Autodesk Inventor part; units mm, degrees
ref_plane "Work Plane2" through (0, 0, 74) normal (0, 0, 1) x (1, 0, 0)
ref_plane "Work Plane3" through (0, 0, 43) normal (0, 0, 1) x (1, 0, 0)
ref_plane "Work Plane6" through (0, 0, 16) normal (0, 0, 1) x (1, 0, 0)
sketch "Sketch1" plane through (0, 0, 0) normal (0, 0, 1) x (1, 0, 0)
  line L0 (-0.2363, 14.3955) -> (15.4637, 14.3955)
  line L1 (15.4637, 14.3955) -> (15.4637, 17.3955)
  line L2 (15.4637, 17.3955) -> (-0.2363, 17.3955)
  line L3 (-0.2363, 17.3955) -> (-0.2363, 14.3955)
  line L4 (15.4637, 14.3955) -> (18.4637, 14.3955)
  line L5 (18.4637, 14.3955) -> (18.4637, -1.3045)
  line L6 (18.4637, -1.3045) -> (15.4637, -1.3045)
  line L7 (15.4637, -1.3045) -> (15.4637, 14.3955)
  line L8 (15.4637, 14.3955) -> (18.4637, 14.3955)
  line L9 (18.4637, 14.3955) -> (18.4637, 17.3955)
  line L10 (18.4637, 17.3955) -> (15.4637, 17.3955)
  line L11 (15.4637, 17.3955) -> (15.4637, 14.3955)
  circle A0 centre (11.9637, 10.8955) radius 2.25
  line L12 (15.4637, 14.3955) -> (8.4637, 14.3955)
  line L13 (8.4637, 14.3955) -> (8.4637, 7.3955)
  line L14 (8.4637, 7.3955) -> (15.4637, 7.3955)
  line L15 (15.4637, 7.3955) -> (15.4637, 14.3955)
  point P0 (0, 0)
  point P1 (11.9637, 7.3955)
  point P2 (8.4637, 10.8955)
  dimension "d2" = 3
  dimension "d3" = 3
  dimension "d9" = 4.5
  dimension "d46" = 7
  dimension "d47" = 7
  dimension "d48" = 15.7
  dimension "d49" = 15.7
extrude "Extrusion1" add sketch "Sketch1" along normal blind 83 contours L3 L2 L1 L0 | L1 L10 L9 L4 | L4 L5 L6 L7
extrude "Extrusion2" add sketch "Sketch1" along normal blind 1.5 contours L0 L7 L14 L13
fillet "Fillet1" radius 3 1 edges at (8.4637, 7.3955, 0.75)
sketch "Sketch3" plane through (-0.2363, 14.3955, 83) normal (0, -1, 0) x (1, 0, 0)
  line L0 (15.7, 0) -> (15.7, -81.5)
  line L1 (0, 0) -> (15.7, 0)
  line L2 (0, -83) -> (0, 0)
  circle A0 centre (6.25, -4) radius 2.25
  line L3 (18.7, -83) -> (0, -83)
  line L4 (0, 0) -> (15.7, 0)
  line L5 (18.7, 0) -> (0, 0)
  line L6 (12.5, 0) -> (12.5, -83) construction
  line L7 (0, -83) -> (0, 0)
  line L8 (12.5, 0) -> (0, 0)
  line L9 (0, -83) -> (8.7, -83)
  line L10 (8.7, -81.5) -> (15.7, -81.5)
  line L11 (8.7, -83) -> (8.7, -81.5)
  point P0 (0.2363, -83)
  point P1 (1.7, -20)
  point P2 (6.25, 0)
  dimension "d12" = 4.5
  dimension "d13" = 4
  dimension "d24" = 12.5
sketch "Sketch4" plane through (15.4637, -1.3045, 83) normal (-1, 0, 0) x (0, 0, 1)
  line L0 (-83, 0) -> (0, 0)
  line L1 (0, 15.7) -> (0, 0)
  line L2 (0, 15.7) -> (-81.5, 15.7)
  circle A0 centre (-4, 6.25) radius 2.25
  line L3 (0, 15.7) -> (0, 0)
  line L4 (-83, 0) -> (-83, 18.7)
  line L5 (0, 15.7) -> (-81.5, 15.7)
  line L6 (0, 12.5) -> (-83, 12.5) construction
  line L7 (0, 12.5) -> (0, 0)
  line L8 (-83, 8.7) -> (-83, 0)
  line L9 (-81.5, 15.7) -> (-81.5, 8.7)
  line L10 (-81.5, 8.7) -> (-83, 8.7)
  point P0 (-83, 1.3045)
  point P1 (-20, 1.7)
  point P2 (0, 6.25)
  point P3 (-83, 15.7)
  dimension "d14" = 4.5
  dimension "d15" = 4
  dimension "d25" = 12.5
extrude "Extrusion4" cut sketch "Sketch3" against normal blind 5 contours A0
extrude "Extrusion5" cut sketch "Sketch4" against normal blind 5 contours A0
sketch "Sketch5" plane through (0, 0, 0) normal (0, 0, 1) x (1, 0, 0)
  line L0 (29.2522, 21.8201) -> (22.8883, 28.184)
  line L1 (22.8883, 28.184) -> (12.2817, 17.5774)
  line L2 (12.2817, 17.5774) -> (18.6456, 11.2135)
  line L3 (18.6456, 11.2135) -> (29.2522, 21.8201)
  line L4 (26.0703, 25.0021) -> (15.4637, 14.3955) construction
  line L5 (23.9489, 16.5168) -> (17.585, 22.8807) construction
  line L6 (15.4637, -1.3045) -> (15.4637, 14.3955)
  line L7 (15.4637, 17.3955) -> (-0.2363, 17.3955)
  line L8 (18.4637, 14.3955) -> (18.4637, -1.3045)
  line L9 (18.4637, 14.3955) -> (18.4637, 17.3955)
  line L10 (18.4637, 17.3955) -> (15.4637, 17.3955)
  circle A0 centre (23.2418, 22.1736) radius 2.25
  line L11 (18.0923, 10.6601) -> (18.6456, 11.2135)
  line L12 (18.6456, 11.2135) -> (12.2817, 17.5774)
  line L13 (12.2817, 17.5774) -> (11.7283, 17.0241)
  line L14 (11.7283, 17.0241) -> (18.0923, 10.6601)
  point P0 (0, 0)
  dimension "d29" = 9
  dimension "d30" = 4.5
  dimension "d31" = 4
  dimension "d32" = 15
  dimension "d56" = 9
extrude "Extrusion6" add sketch "Sketch5" along normal blind 1.5
fillet "Fillet2" radius 2 2 edges at (22.8883, 28.184, 0.75) (29.2522, 21.8201, 0.75)
ref_plane "Work Plane2" through (0, 0, 74) normal (0, 0, 1) x (1, 0, 0)
sketch "Sketch6" plane through (0, 0, 74) normal (0, 0, 1) x (1, 0, 0)
  line L0 (18.4637, -1.3045) -> (18.4637, 17.3955)
  line L1 (18.4637, 17.3955) -> (-0.2363, 17.3955)
  line L2 (-0.2363, 17.3955) -> (-0.2363, 14.3955)
  line L3 (15.4637, -1.3045) -> (18.4637, -1.3045)
  line L4 (-0.2363, 17.3955) -> (-0.2363, 14.3955)
  line L5 (-0.2363, 17.3955) -> (8.4637, 17.3955)
  line L6 (8.4637, 17.3955) -> (8.4637, 14.3955)
  line L7 (8.4637, 14.3955) -> (-0.2363, 14.3955)
  line L8 (-0.2363, 14.3955) -> (-0.2363, 17.3955)
  line L9 (18.4637, -1.3045) -> (15.4637, -1.3045)
  line L10 (15.4637, -1.3045) -> (15.4637, 7.3955)
  line L11 (15.4637, 7.3955) -> (18.4637, 7.3955)
  line L12 (18.4637, 7.3955) -> (18.4637, -1.3045)
  point P0 (0, 0)
  dimension "d45" = 8.7
  dimension "d50" = 7
  dimension "d51" = 7
extrude "Extrusion7" cut sketch "Sketch6" against normal blind 74
ref_plane "Work Plane3" through (0, 0, 43) normal (0, 0, 1) x (1, 0, 0)
ref_plane "Work Plane5" through (0, 0, 39) normal (0, 0, 1) x (1, 0, 0)
sketch "Sketch9" plane through (0, 0, 39) normal (0, 0, 1) x (1, 0, 0)
  line L0 (18.4637, 7.3955) -> (11.4637, 7.3955)
  arc A0 (8.4637, 10.3955) -> (11.4637, 7.3955) centre (11.4637, 10.3955) ccw
  line L1 (8.4637, 10.3955) -> (8.4637, 17.3955)
  line L2 (12.0997, 17.3955) -> (8.4637, 17.3955)
  line L3 (21.4741, 26.7698) -> (12.0997, 17.3955)
  arc A1 (24.3025, 26.7698) -> (21.4741, 26.7698) centre (22.8883, 25.3556) ccw
  line L4 (27.838, 23.2343) -> (24.3025, 26.7698)
  arc A2 (27.838, 20.4059) -> (27.838, 23.2343) centre (26.4238, 21.8201) ccw
  line L5 (18.4637, 11.0315) -> (27.838, 20.4059)
  line L6 (18.4637, 7.3955) -> (18.4637, 11.0315)
  circle A3 centre (23.2418, 22.1736) radius 2.25
  circle A4 centre (11.9637, 10.8955) radius 2.25
  line L7 (12.0997, 17.3955) -> (16.4707, 15.4026)
  line L8 (16.4707, 15.4026) -> (18.4637, 11.0315)
  point P0 (0, 0)
extrude "Extrusion9" add sketch "Sketch9" along normal blind 1.5 contours L8 L7 L3 A1 L4 A2 L5
ref_plane "Work Plane6" through (0, 0, 16) normal (0, 0, 1) x (1, 0, 0)
sketch "Sketch10" plane through (0, 0, 16) normal (0, 0, 1) x (1, 0, 0)
  line L0 (18.4637, 7.3955) -> (11.4637, 7.3955)
  arc A0 (8.4637, 10.3955) -> (11.4637, 7.3955) centre (11.4637, 10.3955) ccw
  line L1 (8.4637, 10.3955) -> (8.4637, 17.3955)
  line L2 (12.0997, 17.3955) -> (8.4637, 17.3955)
  line L3 (21.4741, 26.7698) -> (12.0997, 17.3955)
  arc A1 (24.3025, 26.7698) -> (21.4741, 26.7698) centre (22.8883, 25.3556) ccw
  line L4 (27.838, 23.2343) -> (24.3025, 26.7698)
  arc A2 (27.838, 20.4059) -> (27.838, 23.2343) centre (26.4238, 21.8201) ccw
  line L5 (18.4637, 11.0315) -> (27.838, 20.4059)
  line L6 (18.4637, 7.3955) -> (18.4637, 11.0315)
  circle A3 centre (23.2418, 22.1736) radius 2.25
  circle A4 centre (11.9637, 10.8955) radius 2.25
  line L7 (12.0997, 17.3955) -> (18.4637, 17.3955)
  line L8 (12.0997, 17.3955) -> (16.7869, 15.7187)
  line L9 (18.4637, 17.3955) -> (18.4637, 11.0315)
  line L10 (16.7869, 15.7187) -> (18.4637, 11.0315)
  point P0 (0, 0)
extrude "Extrusion10" add sketch "Sketch10" along normal blind 1.5 contours L9 L7 L3 A1 L4 A2 L5
pattern_linear "Rectangular Pattern2" count 4 spacing 22 along (0, 0, 1) of "Extrusion2", "Fillet1"
ref_plane "Work Plane7" through (0, 0, 63) normal (0, 0, 1) x (1, 0, 0)
sketch "Sketch11" plane through (0, 0, 63) normal (0, 0, 1) x (1, 0, 0)
  arc A0 (27.838, 20.4059) -> (27.838, 23.2343) centre (26.4238, 21.8201) ccw
  line L0 (18.4637, 7.3955) -> (11.4637, 7.3955)
  arc A1 (8.4637, 10.3955) -> (11.4637, 7.3955) centre (11.4637, 10.3955) ccw
  line L1 (8.4637, 10.3955) -> (8.4637, 17.3955)
  line L2 (12.0997, 17.3955) -> (8.4637, 17.3955)
  line L3 (21.4741, 26.7698) -> (12.0997, 17.3955)
  arc A2 (24.3025, 26.7698) -> (21.4741, 26.7698) centre (22.8883, 25.3556) ccw
  line L4 (27.838, 23.2343) -> (24.3025, 26.7698)
  arc A3 (27.838, 20.4059) -> (27.838, 23.2343) centre (26.4238, 21.8201) ccw
  line L5 (18.4637, 11.0315) -> (27.838, 20.4059)
  line L6 (18.4637, 7.3955) -> (18.4637, 11.0315)
  circle A4 centre (23.2418, 22.1736) radius 2.25
  circle A5 centre (11.9637, 10.8955) radius 2.25
  line L7 (18.4637, 11.0315) -> (16.7869, 15.7187)
  line L8 (16.7869, 15.7187) -> (12.0997, 17.3955)
  point P0 (0, 0)
extrude "Extrusion11" add sketch "Sketch11" along normal blind 1.5 contours L5 L7 L8 L3 A2 L4 A0
properties part number "VerticalConnector"
Verification items for the finished model (mm, model axes). A direction names the side the tool comes from. Give positions to 0.01 mm unless a question says otherwise; leave off trailing zeros. Order: outer loops, then holes, each group sorted by start corner. A loop starts at its lowest first (then second) coordinate and runs counter-clockwise, first axis right, second up. Notation, with made-up numbers: (10, -35) -> (30, -35) arc R27 cw to (30, -19) -> close; hole circle Ø6 at (41, 59). An arc over 180 degrees is marked (long way). Use a Markdown table: item, result.
1) Material ranges on probe 1 along Z at (x, y) = (21.5, 19.25); probe 2 along Z at (x, y) = (8.75, 11); probe 3 along X at (y, z) = (14.75, 49), recorded low to high.
Results:
| item | result |
|---|---|
| probe 1 | 0 to 1.5, 16 to 17.5, 39 to 40.5, 63 to 64.5 |
| probe 2 | 0 to 1.5, 22 to 23.5, 44 to 45.5, 66 to 67.5 |
| probe 3 | 8.46 to 18.46 |
2) Section check C-C, the plane y = 25.5. Record the boundary of the cut face in (x, z).
Results:
| item | result |
|---|---|
| outline | (20.2, 0) -> (25.57, 0) -> (25.57, 1.5) -> (20.2, 1.5) -> close; (20.2, 16) -> (25.57, 16) -> (25.57, 17.5) -> (20.2, 17.5) -> close; (20.2, 39) -> (25.57, 39) -> (25.57, 40.5) -> (20.2, 40.5) -> close; (20.2, 63) -> (25.57, 63) -> (25.57, 64.5) -> (20.2, 64.5) -> close |
3) Section check D-D, the plane z = 50.5. Record the boundary of the cut face in (x, y).
Results:
| item | result |
|---|---|
| outline | (8.46, 14.4) -> (15.46, 14.4) -> (15.46, 7.4) -> (18.46, 7.4) -> (18.46, 17.4) -> (8.46, 17.4) -> close |
4) Tool access check on faces 3 (the flat face through (12, 14.396, 34)), 4 (the flat face through (26.09, 24.98, 0.74)). Record the directions out of +Z, -Z, +X, -X, +Y, -Y that give a thin tool (end or side, any length) a straight path to the whole face; none if there is none.
Results:
| item | result |
|---|---|
| face 3 | -X, -Y |
| face 4 | +Z, -Z, +X, +Y |
5) Section check B-B, the plane x = 20.25. Record the boundary of the cut face in (y, z).
Results:
| item | result |
|---|---|
| outline | (12.82, 0) -> (25.55, 0) -> (25.55, 1.5) -> (12.82, 1.5) -> close; (12.82, 16) -> (25.55, 16) -> (25.55, 17.5) -> (12.82, 17.5) -> close; (12.82, 39) -> (25.55, 39) -> (25.55, 40.5) -> (12.82, 40.5) -> close; (12.82, 63) -> (25.55, 63) -> (25.55, 64.5) -> (12.82, 64.5) -> close |
6) Mould release check, pull along Z, two halves, no side actions. Record for faces 1 (the flat face through (23.085, 15.653, 16.74)), 2 (the flat face through (11.9, 13.3, 23.5)): pulls with the +Z half, pulls with the -Z half, needs draft (parallel to the pull), parting line crosses it, or undercut.
Results:
| item | result |
|---|---|
| face 1 | needs draft |
| face 2 | undercut |
7) Depth check by flat-ended pin: pin 1 Ø4 at (x, y) = (11.96, 10.9) entering from -Z; pin 2 Ø2 at (y, z) = (23.5, 39.5) entering from -X; pin 3 Ø7.5 at (y, z) = (14.5, 54.5) entering from -X; pin 4 Ø2 at (x, y) = (10.5, 10.5) entering from +Z. Enter the tip coordinate at first touch or a pass-through.
Results:
| item | result |
|---|---|
| pin 1 | through |
| pin 2 | x = 17.2 |
| pin 3 | x = 8.46 |
| pin 4 | z = 67.5 |
8) Section check A-A, the plane z = 79. Record the boundary of the cut face in (x, y).
Results:
| item | result |
|---|---|
| outline | (-0.24, 14.4) -> (3.76, 14.4) -> (3.76, 17.4) -> (-0.24, 17.4) -> close; (8.26, 14.4) -> (15.46, 14.4) -> (15.46, 7.2) -> (18.46, 7.2) -> (18.46, 17.4) -> (8.26, 17.4) -> close; (15.46, -1.3) -> (18.46, -1.3) -> (18.46, 2.7) -> (15.46, 2.7) -> close |
